Geometry check sheet. Reference: the model listing, model coordinates, mm. Give positions to 0.01 mm unless a question says otherwise; leave off trailing zeros. Loops run counter-clockwise (first coordinate to the right, second up) from the corner with the lowest first, then second, coordinate; pieces in that order, holes last. Notation, with made-up numbers: (30.5, -2) -> (62.5, -2) arc R21 ccw to (62.5, 10) -> close; hole circle Ø10 at (53, 19.25). An arc over 180 degrees is marked (long way). One line per question, with ' | ' between items.
from build123d import *

# Parameters (mm, degrees)
PAD_DEPTH = 10


with BuildPart() as part:
    # Sketch002 → Pad (new body)
    with BuildSketch(Plane.XY):
        with BuildLine():
            ThreePointArc((-18.809847, -3.316572), (16.610979, -9.427904), (-6.796374, 17.849911))
            Line((-6.796374, 34.628607), (-6.796374, 17.849911))
            Line((-6.796374, 34.628607), (-15.115935, 34.628607))
            ThreePointArc((-15.115935, 34.628607), (-19.057395, 32.946654), (-22.522612, 30.425474))
            Line((-22.522612, 30.425474), (-22.522612, 13.051797))
            Line((-22.522612, 13.051797), (-18.809847, -3.316572))
        make_face()
    extrude(amount=PAD_DEPTH)


solid = part.part
Item 1: Scan lines: probe 1 along X at (y, z) = (27, 9.75); probe 2 along Y at (x, z) = (-6.5, 5.75); probe 3 along X at (y, z) = (15, 2). Record each from-to range of solid material in increasing order.
Result:
probe 1: -22.52 to -6.8 | probe 2: -17.96 to 17.96 | probe 3: -22.52 to 11.82
Item 2: Sectioned sample at C-C (x = 0). Record the cut outline in (y, z), plus the area to 3 significant figures.
Result:
outline: (-19.1, 0) -> (19.1, 0) -> (19.1, 10) -> (-19.1, 10) -> close | area: 382 mm2
Item 3: Sectioned sample at A-A (z = 4.5). Record the cut outline in (x, y).
Result:
outline: (-22.52, 13.05) -> (-18.81, -3.32) arc R19.1 ccw (long way) to (-6.8, 17.85) -> (-6.8, 34.63) -> (-15.12, 34.63) arc R19.03 ccw to (-22.52, 30.43) -> close
Item 4: Sectioned sample at B-B (y = 20). Record the cut outline in (x, z).
Result:
outline: (-22.52, 0) -> (-6.8, 0) -> (-6.8, 10) -> (-22.52, 10) -> close
Item 5: Depth check by flat-ended pin: pin 1 Ø5 at (x, z) = (3.5, 1) entering from +Y; pin 2 Ø2 at (y, z) = (-10.5, 6) entering from -X; pin 3 Ø3 at (y, z) = (5.5, 2) entering from -X. Enter the tip coordinate at first touch or a pass-through.
Result:
pin 1: y = 19.07 | pin 2: x = -16.57 | pin 3: x = -21.15
